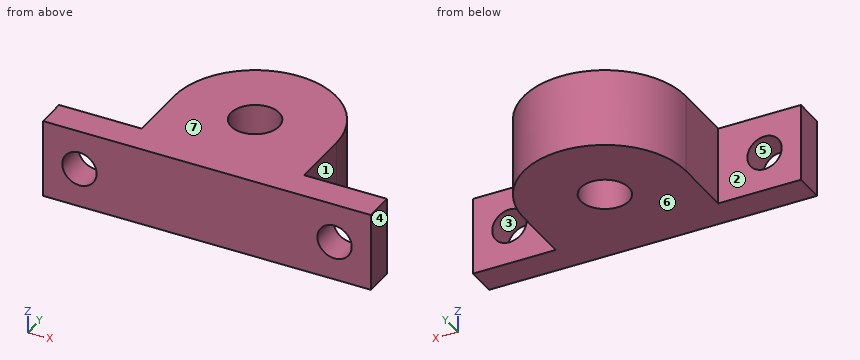
```python
from build123d import *

# Parameters (mm, degrees)
SKETCH1_R           = 4
BOSS_EXTRUDE1_DEPTH = 13
SKETCH2_R           = 2.853745902
CUT_EXTRUDE1_DEPTH  = 13


with BuildPart() as part:
    # Sketch1 → Boss-Extrude1 (new body)
    with BuildSketch(Plane.XY):
        with BuildLine():
            Line((0, 0), (54.5, 0))
            Line((54.5, 0), (54.5, 5))
            Line((54.5, 5), (40.75, 5))
            Line((40.75, 5), (40.75, 15))
            ThreePointArc((40.75, 15), (27.25, 28.5), (13.75, 15))
            Line((13.75, 15), (13.75, 5))
            Line((13.75, 5), (0, 5))
            Line((0, 5), (0, 0))
        make_face()
        with Locations(Location((27.25, 15, 0), (0, 0, 180))):
            Circle(SKETCH1_R, mode=Mode.SUBTRACT)
    extrude(amount=BOSS_EXTRUDE1_DEPTH)

    # Sketch2 → Cut-Extrude1 (cut)
    with BuildSketch(Plane(origin=(0, 5, 0), x_dir=(1, 0, 0), z_dir=(0, 1, 0))):
        with Locations(Location((48.45, -6.5, 0), (0, 0, 180))):
            Circle(SKETCH2_R)
        with Locations(Location((6.05, -6.5, 0), (0, 0, 180))):
            Circle(SKETCH2_R)
    extrude(amount=-CUT_EXTRUDE1_DEPTH, mode=Mode.SUBTRACT)


solid = part.part
```
Input: part model. Units: mm. Frame: model coordinates. Face numbers are marked on the shaded views. A direction names the side the tool comes from. Give positions to 0.01 mm unless a question says otherwise; leave off trailing zeros. Order: outer loops, then holes, each group sorted by start corner. A loop starts at its lowest first (then second) coordinate and runs counter-clockwise, first axis right, second up. Notation, with made-up numbers: (83.25, 86) - (93.25, 86) arc R27 cw to (93.25, 121) - close; hole circle Ø3 at (78, -26.75). An arc over 180 degrees is marked (long way). One line per item, written item: value.
1. Draft query along Z for the marked faces 4, 5, 6 and 7. Return one class per face: released by +Z, released by -Z, zero draft, split by the parting line, or undercut.
Determined:
face 4: zero draft
face 5: undercut
face 6: released by -Z
face 7: released by +Z
2. Cut plane D-D, the plane y = 3.25. Output: boundary loops of the cut face in (x, z).
Determined:
outline: (0, 0) - (54.5, 0) - (54.5, 13) - (0, 13) - close; hole circle Ø5.71 at (6.05, 6.5); hole circle Ø5.71 at (48.45, 6.5)
3. Line query: probe 1 along Z at (x, y) = (48.45, 1.8); probe 2 along X at (y, z) = (2.5, 4); probe 3 along X at (y, z) = (5.5, 2.75). Output: solid intervals per line, ascending.
Determined:
probe 1: 0 to 3.65, 9.35 to 13
probe 2: 0 to 4.67, 7.43 to 47.07, 49.83 to 54.5
probe 3: 13.75 to 40.75
4. Reachability of the marked faces 1, 2 and 3 from +Z, -Z, +X, -X, +Y, -Y: full face, straight path, thin tool, end or side. Return the list, or none.
Determined:
face 1: +Z, -Z, +X, +Y
face 2: +Z, -Z, -X, +Y
face 3: +Y, -Y
5. Cut plane A-A, the plane x = 27.25. Output: boundary loops of the cut face in (y, z).
Determined:
outline: (0, 0) - (11, 0) - (11, 13) - (0, 13) - close; (19, 0) - (28.5, 0) - (28.5, 13) - (19, 13) - close
6. Pin query (flat end, axial travel): pin 1 Ø1 at (x, z) = (25.5, 7) entering from +Y; pin 2 Ø10 at (x, y) = (8.5, 13.5) entering from -Z; pin 3 Ø3 at (x, z) = (42.5, 7) entering from -Y; pin 4 Ø1 at (y, z) = (17, 3.5) entering from +X. Return the tip coordinate at first contact, or that it passes through.
Determined:
pin 1: y = 28.44
pin 2: through
pin 3: y = 0
pin 4: x = 40.67
7. Cut plane B-B, the plane z = 7.5. Output: boundary loops of the cut face in (x, y).
Determined:
outline: (0, 0) - (3.38, 0) - (3.38, 5) - (0, 5) - close; (8.72, 0) - (45.78, 0) - (45.78, 5) - (40.75, 5) - (40.75, 15) arc R13.5 ccw to (13.75, 15) - (13.75, 5) - (8.72, 5) - close; (51.12, 0) - (54.5, 0) - (54.5, 5) - (51.12, 5) - close; hole circle Ø8 at (27.25, 15)
8. Cut plane C-C, the plane y = 11.75. Output: boundary loops of the cut face in (x, z), and give its area (3 significant figures).
Determined:
outline: (13.75, 0) - (24.92, 0) - (24.92, 13) - (13.75, 13) - close; (29.58, 0) - (40.75, 0) - (40.75, 13) - (29.58, 13) - close
area: 290 mm2
